```python
from build123d import *

# Parameters (mm, degrees)
ESQUISSE1_W             = 505
ESQUISSE1_H             = 420
BOSS_EXTRU_1_DEPTH      = 2
ESQUISSE2_R             = 50
ENL_V_MAT_EXTRU_1_DEPTH = 10
ESQUISSE3_R             = 4
ENL_V_MAT_EXTRU_2_DEPTH = 10


with BuildPart() as part:
    # Esquisse1 → Boss.-Extru.1 (new body)
    with BuildSketch(Plane.XY):
        with Locations((0, 2.5)):
            Rectangle(ESQUISSE1_W, ESQUISSE1_H)
    extrude(amount=BOSS_EXTRU_1_DEPTH)

    # Esquisse2 → Enlèv. mat.-Extru.1 (cut)
    with BuildSketch(Plane.XY.offset(2)):
        with Locations((-157.5, 127.5)):
            Circle(ESQUISSE2_R)
    extrude(amount=-ENL_V_MAT_EXTRU_1_DEPTH, mode=Mode.SUBTRACT)

    # Esquisse3 → Enlèv. mat.-Extru.2 (cut)
    with BuildSketch(Plane.XY.offset(2)):
        with Locations((-233.6, 197.5)):
            Circle(ESQUISSE3_R)
        with Locations((-183.6, 197.5)):
            Circle(ESQUISSE3_R)
        with Locations((-61.93, 197.5)):
            Circle(ESQUISSE3_R)
        with Locations((55.17, 197.5)):
            Circle(ESQUISSE3_R)
        with Locations((176.84, 197.5)):
            Circle(ESQUISSE3_R)
        with Locations((226.84, 197.5)):
            Circle(ESQUISSE3_R)
        with Locations((226.84, 67.5)):
            Circle(ESQUISSE3_R)
        with Locations((226.84, -62.5)):
            Circle(ESQUISSE3_R)
        with Locations((226.84, -192.5)):
            Circle(ESQUISSE3_R)
        with Locations((176.84, -192.5)):
            Circle(ESQUISSE3_R)
        with Locations((55.17, -192.5)):
            Circle(ESQUISSE3_R)
        with Locations((-61.93, -192.5)):
            Circle(ESQUISSE3_R)
        with Locations((-183.6, -192.5)):
            Circle(ESQUISSE3_R)
        with Locations((-233.6, -192.5)):
            Circle(ESQUISSE3_R)
        with Locations((-233.6, -62.5)):
            Circle(ESQUISSE3_R)
        with Locations((-233.6, 67.5)):
            Circle(ESQUISSE3_R)
    extrude(amount=-ENL_V_MAT_EXTRU_2_DEPTH, mode=Mode.SUBTRACT)


solid = part.part
```
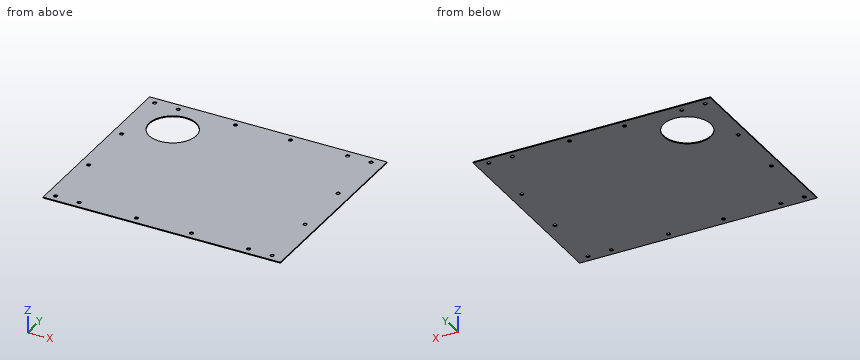
Can you work these out from the model? Positions are in its coordinate system, mm. Give positions to 0.01 mm unless a question says otherwise; leave off trailing zeros. Order: outer loops, then holes, each group sorted by start corner. A loop starts at its lowest first (then second) coordinate and runs counter-clockwise, first axis right, second up. Notation, with made-up numbers: (-26, 19.5) - (10, 19.5) arc R19 cw to (10, 42.5) - close; hole circle Ø8 at (71, 40). An arc over 180 degrees is marked (long way). Use a Markdown table: item, result. Add a question column.
Q1. If we section it at B-B on x = -139: Write out the boundary of the cut face in (y, z), plus the area to 3 significant figures.
Q2. I'm going to push a flat-ended pin straight in: pin 1 (5 mm diameter, centred on x = -183.6, y = 197.5, fed in from +Z). Where does the tip first touch, or does it pass through?
Q3. If we section it at A-A on z = 0.8: Count the separate pieces of the cut face and the enclosed holes in it, plus the area to 3 significant figures.
Q4. Please list where these lines run through material, in increasing order: line 1 along Y through (x, z) = (-61.93, 0.55); line 2 along Y through (x, z) = (-183.6, 0.6); line 3 along Y through (x, z) = (-233.6, 1.1).
Answers follow:
| question | item | result |
|---|---|---|
| 1 | outline | (-207.5, 0) - (81.05, 0) - (81.05, 2) - (-207.5, 2) - close; (173.95, 0) - (212.5, 0) - (212.5, 2) - (173.95, 2) - close |
| 1 | area | 654 mm^2 |
| 2 | pin 1 | passes through |
| 3 | separate pieces | 1 |
| 3 | enclosed holes | 17 |
| 3 | area | 203,000 mm^2 |
| 4 | line 1 | y = -207.5 to -196.5, -188.5 to 193.5, 201.5 to 212.5 |
| 4 | line 2 | y = -207.5 to -196.5, -188.5 to 84.85, 170.15 to 193.5, 201.5 to 212.5 |
| 4 | line 3 | y = -207.5 to -196.5, -188.5 to -66.5, -58.5 to 63.5, 71.5 to 193.5, 201.5 to 212.5 |
